from build123d import *

# Parameters (mm, degrees)
CROQUIS1_W                 = 118
CROQUIS1_H                 = 84.6
SALIENTE_EXTRUIR1_DEPTH    = 36
CROQUIS2_W                 = 36
CROQUIS2_H                 = 74.6
CORTAR_EXTRUIR1_DEPTH      = 120
CORTAR_EXTRUIR3_DEPTH      = 110.243581047
SALIENTE_EXTRUIR2_DEPTH    = 84.6
CROQUIS8_W                 = 160.5
CROQUIS8_H                 = 84.6
SALIENTE_EXTRUIR3_DEPTH    = 5
CROQUIS9_W                 = 41
CROQUIS9_H                 = 84.6
SALIENTE_EXTRUIR4_DEPTH    = 5
CROQUIS10_W                = 5
CROQUIS10_H                = 84.6
SALIENTE_EXTRUIR5_DEPTH    = 5
REDONDEO2_R                = 10
REDONDEO3_R                = 2
REDONDEO4_R                = 2
CROQUIS18_W                = 165.5
CROQUIS18_H                = 84.6
SALIENTE_EXTRUIR9_DEPTH    = 6
CORTAR_EXTRUIR6_DEPTH      = 120.584865263
CORTAR_EXTRUIR6_DEPTH_BACK = 120.584865263
CROQUIS11_R                = 6
CROQUIS16_R                = 6
SALIENTE_EXTRUIR8_DEPTH    = 5
CROQUIS17_R                = 3
CORTAR_EXTRUIR7_DEPTH      = 120.584865302


with BuildPart() as part:
    # Croquis1 → Saliente-Extruir1 (new body)
    with BuildSketch(Plane.XY):
        Rectangle(CROQUIS1_W, CROQUIS1_H)
    extrude(amount=SALIENTE_EXTRUIR1_DEPTH)

    # Croquis2 → Cortar-Extruir1 (cut)
    with BuildSketch(Plane(origin=(59, 0, 0), x_dir=(0, 0, -1), z_dir=(1, 0, 0))):
        with Locations((-18, 0)):
            Rectangle(CROQUIS2_W, CROQUIS2_H)
    extrude(amount=-CORTAR_EXTRUIR1_DEPTH, mode=Mode.SUBTRACT)


with BuildPart() as cortar_extruir1_piece_1:
    # of the separate pieces the step leaves, piece 1, a body of its own (cortar_extruir1_pieces)
    add(part.part.solids().sort_by_distance((-59, -42.3, 0))[0])


with BuildPart() as cortar_extruir1_piece_2:
    # of the separate pieces the step leaves, piece 2, a body of its own (cortar_extruir1_pieces)
    add(part.part.solids().sort_by_distance((-59, 42.3, 0))[0])


with BuildPart() as cortar_extruir3_tool:
    # Croquis6 → Cortar-Extruir3 (new, through all)
    with BuildSketch(Plane.XZ.offset(42.3)):
        with BuildLine():
            Line((-59, 0), (-59, 36))
            Line((-59, 36), (0, 36))
            ThreePointArc((0, 36), (-33.535731191, 24.614115008), (-59, 0))
        make_face()
    extrude(amount=-CORTAR_EXTRUIR3_DEPTH)


with BuildPart() as cortar_extruir1_piece_1_1:
    add(cortar_extruir1_piece_1.part)

    # Cortar-Extruir3: cut by cortar_extruir3_tool
    add(cortar_extruir3_tool.part, mode=Mode.SUBTRACT)



with BuildPart() as cortar_extruir1_piece_2_1:
    add(cortar_extruir1_piece_2.part)

    # Cortar-Extruir3: cut by cortar_extruir3_tool
    add(cortar_extruir3_tool.part, mode=Mode.SUBTRACT)


with BuildPart() as body_3:
    # Croquis7 → Saliente-Extruir2 (new, through all)
    with BuildSketch(Plane.XZ.offset(-42.3)):
        with BuildLine():
            Line((-59, 0), (-59, 36))
            Line((-59, 36), (0, 36))
            ThreePointArc((0, 36), (-33.535731191, 24.614115008), (-59, 0))
        make_face()
    extrude(amount=SALIENTE_EXTRUIR2_DEPTH)


with BuildPart() as cortar_extruir1_piece_1_2:
    add(cortar_extruir1_piece_1_1.part)

    add(cortar_extruir1_piece_2_1.part)  # Saliente-Extruir3 merges Cortar-Extruir1 piece 2

    add(body_3.part)  # Saliente-Extruir3 merges body 3
    # Croquis8 → Saliente-Extruir3 (add)
    with BuildSketch(Plane.XY.offset(36)):
        with Locations((21.25, 0)):
            Rectangle(CROQUIS8_W, CROQUIS8_H)
    extrude(amount=SALIENTE_EXTRUIR3_DEPTH)

    # Croquis9 → Saliente-Extruir4 (add)
    with BuildSketch(Plane.ZY.offset(59)):
        with Locations((20.5, 0)):
            Rectangle(CROQUIS9_W, CROQUIS9_H)
    extrude(amount=SALIENTE_EXTRUIR4_DEPTH)

    # Croquis10 → Saliente-Extruir5 (add)
    with BuildSketch(Plane(origin=(0, 0, 36), x_dir=(-1, 0, 0), z_dir=(0, 0, -1))):
        with Locations((-99, 0)):
            Rectangle(CROQUIS10_W, CROQUIS10_H)
    extrude(amount=SALIENTE_EXTRUIR5_DEPTH)

    # Redondeo2
    redondeo2_edges = [cortar_extruir1_piece_1_2.edges().sort_by_distance(p)[0] for p in [
        (59, -39.8, 36),
        (59, -39.8, 0),
        (59, 39.8, 36),
        (59, 39.8, 0),
    ]]
    fillet(redondeo2_edges, radius=REDONDEO2_R)

    # Redondeo3
    redondeo3_edges = [cortar_extruir1_piece_1_2.edges().sort_by_distance(p)[0] for p in [
        (101.5, 0, 31),
        (99, -42.3, 31),
        (99, 42.3, 31),
    ]]
    fillet(redondeo3_edges, radius=REDONDEO3_R)

    # Redondeo4
    redondeo4_edges = [cortar_extruir1_piece_1_2.edges().sort_by_distance(p)[0] for p in [
        (-7.5, -42.3, 0),
        (-64, 0, 0),
        (82.75, 42.3, 36),
        (82.75, -42.3, 36),
        (59, -42.3, 18),
        (-7.5, 42.3, 0),
        (56.071067812, -42.3, 2.928932188),
        (59, 42.3, 18),
        (56.071067812, 42.3, 2.928932188),
        (61.928932188, -42.3, 33.071067812),
        (61.928932188, 42.3, 33.071067812),
    ]]
    fillet(redondeo4_edges, radius=REDONDEO4_R)

    # Croquis18 → Saliente-Extruir9 (add)
    with BuildSketch(Plane.XY.offset(41)):
        with Locations((18.75, 0)):
            Rectangle(CROQUIS18_W, CROQUIS18_H)
    extrude(amount=SALIENTE_EXTRUIR9_DEPTH)

    # Croquis11 → Cortar-Extruir6 (cut, two sides: drawn at the far end of the back side and taken through both)
    with BuildSketch(Plane.XY.offset(47).offset(-CORTAR_EXTRUIR6_DEPTH_BACK)):
        with Locations((-36, 13.25)):
            Circle(CROQUIS11_R)
        with Locations((-9.5, 13.25)):
            Circle(CROQUIS11_R)
        with Locations((-9.5, -13.25)):
            Circle(CROQUIS11_R)
        with Locations((-36, -13.25)):
            Circle(CROQUIS11_R)
    extrude(amount=CORTAR_EXTRUIR6_DEPTH + CORTAR_EXTRUIR6_DEPTH_BACK, mode=Mode.SUBTRACT)

    # Croquis16 → Saliente-Extruir8 (add)
    with BuildSketch(Plane.XY.offset(47)):
        with Locations((-9.5, 13.25)):
            Circle(CROQUIS16_R)
        with Locations((-36, -13.25)):
            Circle(CROQUIS16_R)
        with Locations((-9.5, -13.25)):
            Circle(CROQUIS16_R)
        with Locations((-36, 13.25)):
            Circle(CROQUIS16_R)
    extrude(amount=-SALIENTE_EXTRUIR8_DEPTH)

    # Croquis17 → Cortar-Extruir7 (cut, through all)
    with BuildSketch(Plane.XY.offset(47)):
        with Locations((-9.5, 13.25)):
            Circle(CROQUIS17_R)
        with Locations((-36, 13.25)):
            Circle(CROQUIS17_R)
        with Locations((-9.5, -13.25)):
            Circle(CROQUIS17_R)
        with Locations((-36, -13.25)):
            Circle(CROQUIS17_R)
    extrude(amount=-CORTAR_EXTRUIR7_DEPTH, mode=Mode.SUBTRACT)


solid = cortar_extruir1_piece_1_2.part
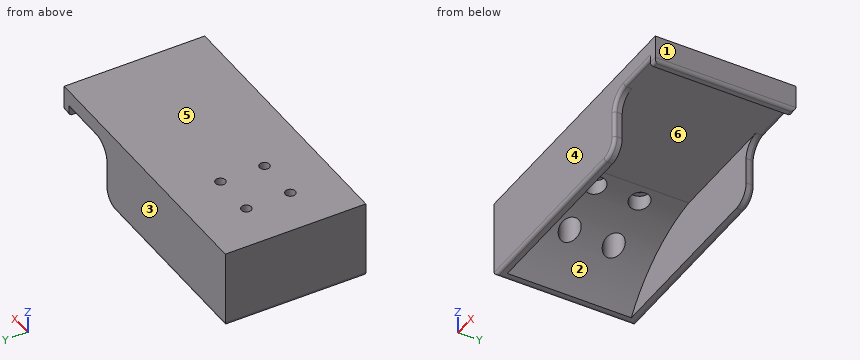
Verification items for the finished model (mm, model axes). Face numbers are marked on the shaded views. A direction names the side the tool comes from. Coordinates: 2 decimals unless noted, no trailing zeros. Order: outer loops, then holes, each group sorted by start corner. A loop starts at its lowest first (then second) coordinate and runs counter-clockwise, first axis right, second up.
Item 1: Section check C-C, the plane y = -2. Enter the section's corners in (x, z), then the cut area to 3 significant figures.
Filled in:
outline: (-64, 2) arc R2 ccw to (-62, 0) - (-59, 0) arc R80.94 cw to (0, 36) - (96.5, 36) - (96.5, 31) - (99.5, 31) arc R2 ccw to (101.5, 33) - (101.5, 47) - (-64, 47) - close
area: 2,730 mm2
Item 2: Material ranges on L1, parallel to Y at x = -9.5, z = 43.35; L2, parallel to X at y = -13, z = 43; L3, parallel to Y at x = 28, z = 26, recorded low to high.
Filled in:
L1: y = -42.3 to -16.25, -10.25 to 10.25, 16.25 to 42.3
L2: x = -64 to -38.99, -33.01 to -12.49, -6.51 to 101.5
L3: y = -42.3 to -37.3, 37.3 to 42.3
Item 3: Release check for a two-part mould opening along Y. For the marked faces 1, 2, 3 and 4 record: +Y half, -Y half, draft (parallel to the pull), parting line (faces both ways), or undercut.
Filled in:
face 1: draft
face 2: undercut
face 3: +Y half
face 4: -Y half
Item 4: Section check D-D, the plane y = -13.25. Enter the section's corners in (x, z), then the cut area to 3 significant figures.
Filled in:
outline: (-64, 2) arc R2 ccw to (-62, 0) - (-59, 0) arc R80.94 cw to (-42, 18.68) - (-42, 42) - (-39, 42) - (-39, 47) - (-64, 47) - close; (-33, 42) - (-30, 42) - (-30, 26.65) arc R80.94 cw to (-15.5, 32.78) - (-15.5, 42) - (-12.5, 42) - (-12.5, 47) - (-33, 47) - close; (-6.5, 42) - (-3.5, 42) - (-3.5, 35.55) arc R80.94 cw to (0, 36) - (96.5, 36) - (96.5, 31) - (99.5, 31) arc R2 ccw to (101.5, 33) - (101.5, 47) - (-6.5, 47) - close
area: 2,340 mm2
Item 5: Depth check by flat-ended pin: pin 1 (19 mm diameter, centred on x = -9.5, y = -13.25, fed in from -Z); pin 2 (19 mm diameter, centred on x = -36, y = 13.25, fed in from +Z); pin 3 (1.5 mm diameter, centred on x = 97.5, y = -5, fed in from -Z); pin 4 (12 mm diameter, centred on x = 31, y = 18.5, fed in from -Z). Enter the tip coordinate at first touch or a pass-through.
Filled in:
pin 1: stops at z = 31.6
pin 2: stops at z = 47
pin 3: stops at z = 31
pin 4: stops at z = 36
Item 6: Section check B-B, the plane x = -36. Enter the section's corners in (y, z), then the cut area to 3 significant figures.
Filled in:
outline: (-42.3, 2) arc R2 ccw to (-40.3, 0) - (-37.3, 0) - (-37.3, 23.05) - (-19.25, 23.05) - (-19.25, 42) - (-16.25, 42) - (-16.25, 47) - (-42.3, 47) - close; (-10.25, 42) - (-7.25, 42) - (-7.25, 23.05) - (7.25, 23.05) - (7.25, 42) - (10.25, 42) - (10.25, 47) - (-10.25, 47) - close; (16.25, 42) - (19.25, 42) - (19.25, 23.05) - (37.3, 23.05) - (37.3, 0) - (40.3, 0) arc R2 ccw to (42.3, 2) - (42.3, 47) - (16.25, 47) - close
area: 1,740 mm2
Item 7: Section check A-A, the plane z = 40. Enter the section's corners in (x, y).
Filled in:
outline: (-64, -42.3) - (101.5, -42.3) - (101.5, 42.3) - (-64, 42.3) - close; hole circle Ø12 at (-36, -13.25); hole circle Ø12 at (-36, 13.25); hole circle Ø12 at (-9.5, -13.25); hole circle Ø12 at (-9.5, 13.25)
Item 8: Access from +Z, -Z, +X, -X, +Y, -Y to the whole of each face (thin tool, end or side, straight path). Record for the marked faces 5 and 6.
Filled in:
face 5: +Z, +X, -X, +Y, -Y
face 6: -Z
